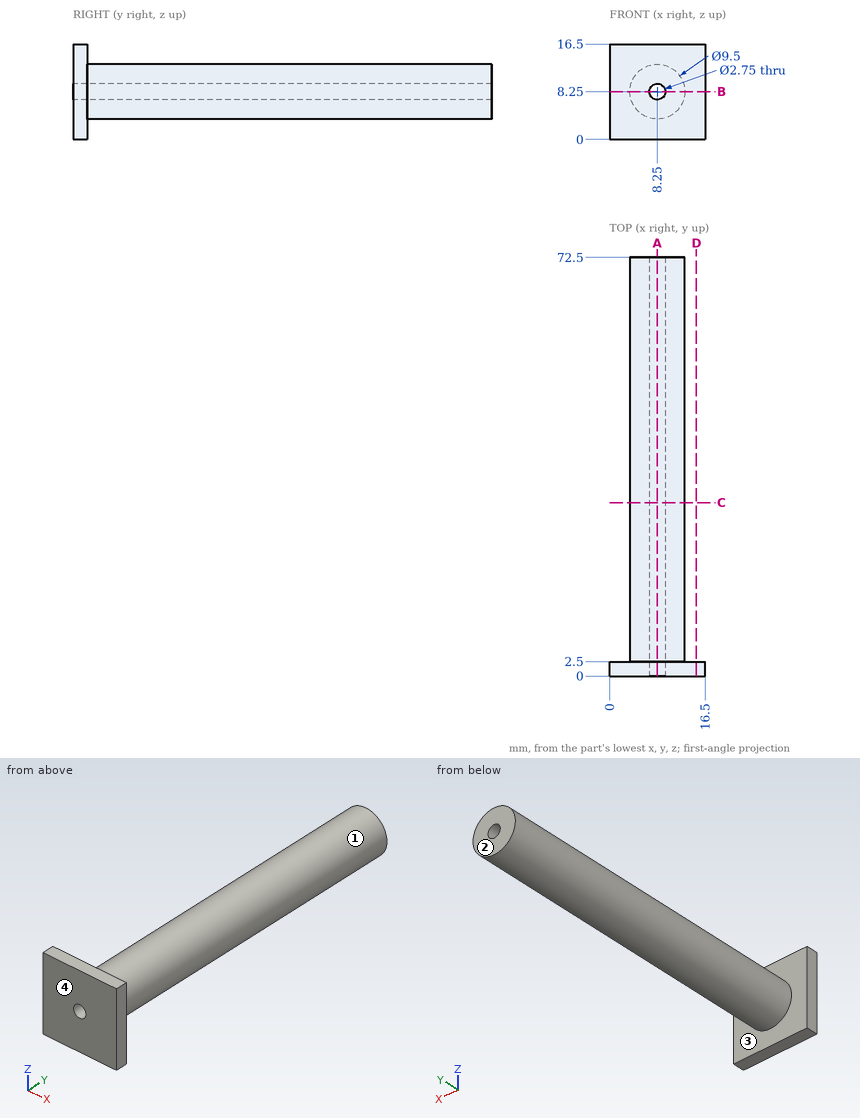
Print and shaded views of the part. All mm, measured from the part's lowest x, y and z. A direction names the side the tool comes from. Coordinates: 2 decimals unless noted, no trailing zeros. Order: outer loops, then holes, each group sorted by start corner. A loop starts at its lowest first (then second) coordinate and runs counter-clockwise, first axis right, second up.
(1) Slice it at A-A, the plane x = 8.25. Write the cut outline in (y, z) (3 decimals), and give its area (3 significant figures).
Check sheet entries:
outline: (0, 0) - (2.5, 0) - (2.5, 3.5) - (72.5, 3.5) - (72.5, 6.875) - (0, 6.875) - close; (0, 9.625) - (72.5, 9.625) - (72.5, 13) - (2.5, 13) - (2.5, 16.5) - (0, 16.5) - close
area: 507 mm2
(2) Probe L1, parallel to Z at x = 8.25, y = 34 (3 decimals); L2, parallel to Y at x = 1.5, z = 4.5. List the from-to ranges inside material, lowest first.
Check sheet entries:
L1: z = 3.5 to 6.875, 9.625 to 13
L2: y = 0 to 2.5
(3) Pin check, flat tips, straight feed: pin 1 Ø8 at (y, z) = (61, 14) entering from +X; pin 2 Ø2 at (x, z) = (8.25, 8.25) entering from +Y; pin 3 Ø5 at (x, y) = (4.5, 39.5) entering from -Z; pin 4 Ø8 at (y, z) = (24.5, 12.5) entering from -X. Stop position of each tip, or through.
Check sheet entries:
pin 1: stops at x = 12.67
pin 2: passes through
pin 3: stops at z = 3.67
pin 4: stops at x = 3.51
(4) Pull direction Z, two halves, no side cores. Call the marked faces 1 and 2: pulls with the +Z half, pulls with the -Z half, needs draft (parallel to the pull), parting line crosses it, or undercut.
Check sheet entries:
face 1: parting line crosses it
face 2: needs draft
(5) Slice it at D-D, the plane x = 15. Write the cut outline in (y, z), and give its area (4 significant figures).
Check sheet entries:
outline: (0, 0) - (2.5, 0) - (2.5, 16.5) - (0, 16.5) - close
area: 41.25 mm2
(6) Slice it at C-C, the plane y = 30. Write the cut outline in (x, z) (3 decimals).
Check sheet entries:
outline: circle Ø9.5 at (8.25, 8.25); hole circle Ø2.75 at (8.25, 8.25)
(7) Tool access for the marked faces 3 and 4: list every direction of +Z, -Z, +X, -X, +Y, -Y with a clear straight run to the whole face (end or side of a thin tool).
Check sheet entries:
face 3: +Y
face 4: +Z, -Z, +X, -X, -Y
(8) Slice it at B-B, the plane z = 8.25. Write the cut outline in (x, y) (3 decimals), and give its area (3 significant figures).
Check sheet entries:
outline: (0, 0) - (6.875, 0) - (6.875, 72.5) - (3.5, 72.5) - (3.5, 2.5) - (0, 2.5) - close; (9.625, 0) - (16.5, 0) - (16.5, 2.5) - (13, 2.5) - (13, 72.5) - (9.625, 72.5) - close
area: 507 mm2
